The model under review builds one solid part; all positions refer to its coordinate system, in mm. A direction names the side the tool comes from. Give positions to 0.01 mm unless a question says otherwise; leave off trailing zeros. Order: outer loops, then holes, each group sorted by start corner. A loop starts at its lowest first (then second) coordinate and runs counter-clockwise, first axis right, second up. Notation, with made-up numbers: (32.25, 24.5) - (64.25, 24.5) arc R8 ccw to (64.25, 34.5) - close; hole circle Ø7 at (4.25, 10). An arc over 180 degrees is marked (long way). Use CSV: the item, a comma, the result in double quotes. Start each with the question number.
```python
from build123d import *

# Parameters (mm, degrees)
F1_R      = 2.4765
F2_DEPTH  = 20.32
F3_W      = 58.3565
F3_H      = 3.556
F3_W_2    = 47.03826
F4_DEPTH  = 131.572
F5_R      = 3.175
F6_W      = 62.404111
F6_H      = 27.47877
F7_DEPTH  = 32.385
F8_W      = 49.20488
F8_H      = 17.78
F8_W_2    = 58.3565
F8_W_3    = 107.56138
F9_DEPTH  = 19.05
F10_R     = 4.191
F11_DEPTH = 130.175


with BuildPart() as f2:
    # F1 (on Top) → F2 (new body)
    with BuildSketch(Plane.XY):
        Polygon((68.5165, 50.8), (0, 50.8), (-68.5165, 50.8), (-68.5165, 0), (-68.5165, -50.8), (0, -50.8), (68.5165, -50.8), (68.5165, 0), align=None)
        with Locations((-60.8965, -43.18)):
            Circle(F1_R, mode=Mode.SUBTRACT)
        with Locations((60.8965, -43.18)):
            Circle(F1_R, mode=Mode.SUBTRACT)
        with Locations((-60.8965, 43.18)):
            Circle(F1_R, mode=Mode.SUBTRACT)
        with Locations((60.8965, 43.18)):
            Circle(F1_R, mode=Mode.SUBTRACT)
    extrude(amount=F2_DEPTH)

    # F3 (on face) → F4 (cut)
    with BuildSketch(Plane(origin=(0, 50.8, 0), x_dir=(-1, 0, 0), z_dir=(0, 1, 0))):
        with Locations((-29.17825, 18.542)):
            Rectangle(F3_W, F3_H)
        with Locations((23.51913, 18.542)):
            Rectangle(F3_W_2, F3_H)
    extrude(amount=-F4_DEPTH, mode=Mode.SUBTRACT)

    # F5
    f5_edges = [f2.edges().sort_by_distance(p)[0] for p in [
        (68.5165, 50.8, 10.16),
        (-68.5165, 50.8, 10.16),
        (-68.5165, -50.8, 10.16),
        (68.5165, -50.8, 10.16),
    ]]
    fillet(f5_edges, radius=F5_R)

    # F6 (on offset) → F7 (cut, symmetric)
    with BuildSketch(Plane.YZ.offset(4.826)):
        with Locations((31.202056, 13.739385)):
            Rectangle(F6_W, F6_H)
    extrude(amount=F7_DEPTH, both=True, mode=Mode.SUBTRACT)

    # F8 (on face) → F9 (cut)
    with BuildSketch(Plane.XY.offset(20.32)):
        with Locations((-24.60244, 29.21)):
            Rectangle(F8_W, F8_H)
        with Locations((29.17825, 29.21)):
            Rectangle(F8_W_2, F8_H)
        with Locations((4.57581, -29.21)):
            Rectangle(F8_W_3, F8_H)
    extrude(amount=-F9_DEPTH, mode=Mode.SUBTRACT)

    # F10 (on face) → F11 (cut)
    with BuildSketch(Plane(origin=(-68.5165, 0, 0), x_dir=(0, -1, 0), z_dir=(-1, 0, 0))):
        with Locations((-29.21, 10.19175)):
            Circle(F10_R)
        with Locations((29.21, 10.19175)):
            Circle(F10_R)
    extrude(amount=-F11_DEPTH, mode=Mode.SUBTRACT)


solid = f2.part
```
1. Consider section B-B (y = -43.18). Give the boundary of the cut face in (x, z).
2. Clearance check with flat-ended pins moving along their axes: pin 1 (9 mm diameter, centred on x = -39.5, y = 27, fed in from +Z); pin 2 (6.5 mm diameter, centred on x = 45.5, y = 44, fed in from +Z); pin 3 (5 mm diameter, centred on y = -29.21, z = 10.19, fed in from -X); pin 4 (4.5 mm diameter, centred on x = 60.9, y = 43.18, fed in from -Z). State where each tip first meets the part, or that it passes through.
3. Tool access review of faces 1 (the face through (4, -29, 1.27)), 2 (the face through (37.211, 19, 8)), 3 (the face through (-47.038, 0, 19)), 4 (the face through (-58.996, -33.207, 11.451)): name each direction out of +Z, -Z, +X, -X, +Y, -Y from which nothing blocks a thin tool from reaching the whole face with its end or side.
4. Mouldability with a two-part tool opening along Y and no side actions: class faces 5 (the face through (-1, -50.8, 8)), 6 (the face through (-1, -11, 0)), 7 (the face through (-58.534, 43.924, 10.018)) as pulls with the +Y half, pulls with the -Y half, needs draft (parallel to the pull), parting line crosses it, or undercut.
5. Consider section A-A (y = 6.5). Give the boundary of the cut face in (x, z).
6. To check wall thickness, follow L1, parallel to Y at x = -41, z = 8.5; L2, parallel to Z at x = -57, y = 29.21; L3, parallel to X at y = 7.5, z = 5.5. State the ranges of each line that lie inside material, in increasing order. Write a range as [from, to].
7. Consider section D-D (x = -6). Give the boundary of the cut face in (y, z).
8. Consider section C-C (y = 43.18). Give the boundary of the cut face in (x, z).
Answers follow:
1,outline,"(-68.52, 0) - (-63.37, 0) - (-63.37, 20.32) - (-68.52, 20.32) - close; (-58.42, 0) - (58.42, 0) - (58.42, 20.32) - (58.36, 20.32) - (58.36, 16.76) - (-47.04, 16.76) - (-47.04, 20.32) - (-58.42, 20.32) - close; (63.37, 0) - (68.52, 0) - (68.52, 20.32) - (63.37, 20.32) - close"
2,pin 1,"stops at z = 1.27"
2,pin 2,"stops at z = 16.76"
2,pin 3,"stops at x = 61.66"
2,pin 4,"passes through"
3,face 1,"+Z"
3,face 2,"+Z, -Z, +Y"
3,face 3,"+Z, +Y, -Y"
3,face 4,"-X"
4,face 5,"pulls with the -Y half"
4,face 6,"needs draft"
4,face 7,"undercut"
5,outline,"(-68.52, 0) - (-27.56, 0) - (-27.56, 16.76) - (-47.04, 16.76) - (-47.04, 20.32) - (-68.52, 20.32) - close; (37.21, 0) - (68.52, 0) - (68.52, 20.32) - (58.36, 20.32) - (58.36, 16.76) - (37.21, 16.76) - close"
6,L1,"y = [-50.8, -38.1], [-20.32, 20.32], [38.1, 50.8]"
6,L2,"z = [0, 6], [14.38, 20.32]"
6,L3,"x = [-68.52, -27.56], [37.21, 68.52]"
7,outline,"(-50.8, 0) - (0, 0) - (0, 16.76) - (-20.32, 16.76) - (-20.32, 1.27) - (-38.1, 1.27) - (-38.1, 16.76) - (-50.8, 16.76) - close"
8,outline,"(-68.52, 0) - (-63.37, 0) - (-63.37, 20.32) - (-68.52, 20.32) - close; (-58.42, 0) - (-27.56, 0) - (-27.56, 16.76) - (-47.04, 16.76) - (-47.04, 20.32) - (-58.42, 20.32) - close; (37.21, 0) - (58.42, 0) - (58.42, 20.32) - (58.36, 20.32) - (58.36, 16.76) - (37.21, 16.76) - close; (63.37, 0) - (68.52, 0) - (68.52, 20.32) - (63.37, 20.32) - close"
